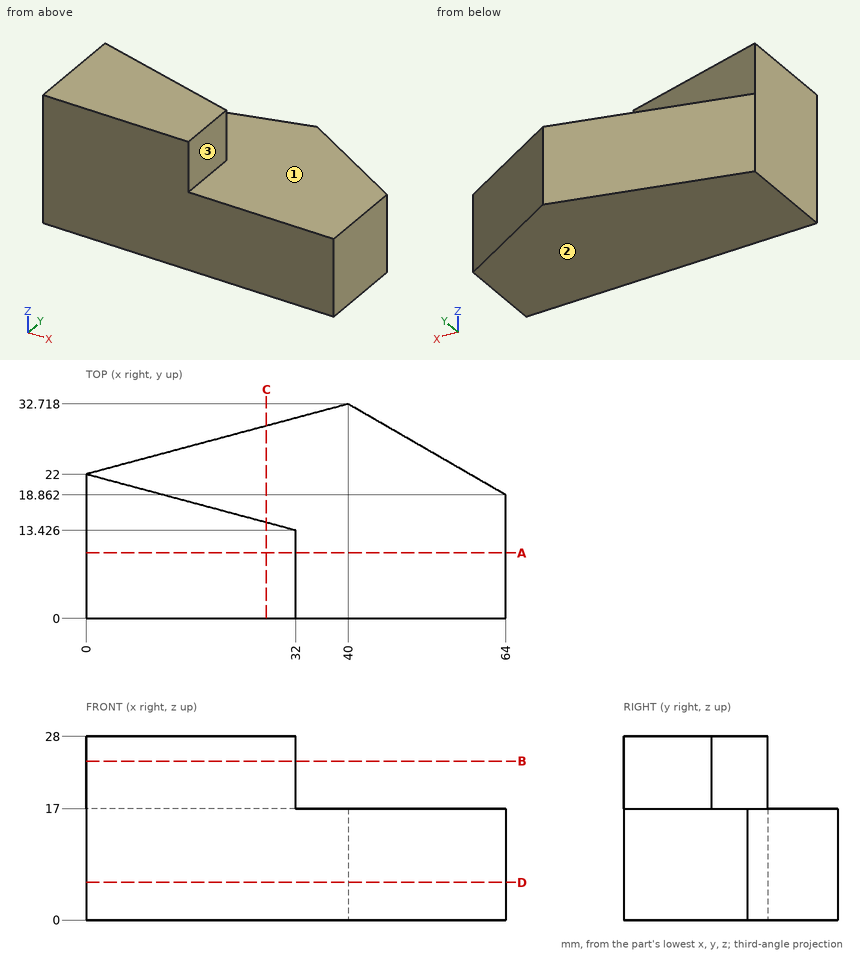
The drawing under review shows one solid part. Ordinate dimensions are in mm from its lowest x, y, z. A direction names the side the tool comes from. Round coordinates to 2 decimals unless told otherwise and drop trailing zeros. Loops run counter-clockwise (first coordinate to the right, second up) from the corner with the lowest first, then second, coordinate; pieces in that order, holes last. Notation, with made-up numbers: (-16.75, 39.5) - (18.25, 39.5) arc R30 cw to (18.25, 74.5) - close; hole circle Ø7 at (-8, -2). An arc over 180 degrees is marked (long way). Put each result on its own line as item: value. Start each with the question number.
1. Consider section D-D on z = 5.75. State the section outline as (x, y) points.
2. Consider section B-B on z = 24.25. State the section outline as (x, y) points (1 decimal).
3. For probe 1 along Z at (x, y) = (26, 16); probe 2 along X at (y, z) = (8.5, 17.25); probe 3 along Y at (x, z) = (26, 21.25), list the stretches that pass through material, from the lowest coordinate up. Write a range as [from, to].
4. Insertion check: P1, Ø3, axis at x = 54, z = 13, coming from the +Y side; P2, Ø2, axis at x = 22, z = 15.5, coming from the +Y side; P3, Ø9, axis at y = 7, z = 23, coming from the +X side. Each pin has a flat end and moves straight along its axis. Give the tip position at first contact, or say it passes through.
5. For the marked faces 1, 2 and 3, list the 3-axis set-ups (+Z, -Z, +X, -X, +Y, -Y) from which the entire face can be reached by the end or side of a thin tool; tool diameter is ignored.
6. Consider section A-A on y = 10. State the section outline as (x, z) points, plus the area to 3 significant figures.
7. Consider section C-C on x = 27.5. State the section outline as (y, z) points, plus the area to 3 significant figures.
Result sheet:
1. outline: (0, 0) - (64, 0) - (64, 18.86) - (40, 32.72) - (0, 22) - close
2. outline: (0, 0) - (32, 0) - (32, 13.4) - (0, 22) - close
3. probe 1: [0, 17]
3. probe 2: [0, 32]
3. probe 3: [0, 15.03]
4. P1: y = 25.5
4. P2: y = 28.16
4. P3: x = 32
5. face 1: +Z, +X, +Y
5. face 2: -Z, +X, -X, +Y, -Y
5. face 3: +Z, +X, +Y, -Y
6. outline: (0, 0) - (64, 0) - (64, 17) - (32, 17) - (32, 28) - (0, 28) - close
6. area: 1,440 mm^2
7. outline: (0, 0) - (29.37, 0) - (29.37, 17) - (14.63, 17) - (14.63, 28) - (0, 28) - close
7. area: 660 mm^2
